from build123d import *

# Parameters (mm, degrees)
SKETCH1_W           = 25
SKETCH1_H           = 23.9
SKETCH1_R           = 1
BOSS_EXTRUDE1_DEPTH = 0.95
SKETCH2_W           = 7.5
SKETCH2_H           = 5
BOSS_EXTRUDE2_DEPTH = 1.45
SKETCH3_W           = 8
SKETCH3_H           = 8
BOSS_EXTRUDE3_DEPTH = 4.4
SKETCH4_W           = 8
SKETCH4_H           = 8
SKETCH4_R           = 3.75
CUT_EXTRUDE1_DEPTH  = 0.9
SKETCH5_R           = 2.775
CUT_EXTRUDE2_DEPTH  = 3.9
BOSS_EXTRUDE4_DEPTH = 6
BOSS_EXTRUDE5_DEPTH = 2.8


with BuildPart() as part:
    # Sketch1 → Boss-Extrude1 (new body)
    with BuildSketch(Plane.XY):
        with Locations((12.5, 11.95)):
            Rectangle(SKETCH1_W, SKETCH1_H)
        with Locations((23, 9.35)):
            Circle(SKETCH1_R, mode=Mode.SUBTRACT)
        with Locations((2, 9.35)):
            Circle(SKETCH1_R, mode=Mode.SUBTRACT)
        with Locations((23, 21.85)):
            Circle(SKETCH1_R, mode=Mode.SUBTRACT)
        with Locations((2, 21.85)):
            Circle(SKETCH1_R, mode=Mode.SUBTRACT)
    extrude(amount=BOSS_EXTRUDE1_DEPTH)

    # Sketch2 → Boss-Extrude2 (add)
    with BuildSketch(Plane.XY.offset(0.95)):
        with Locations((12.5, 19.2)):
            Rectangle(SKETCH2_W, SKETCH2_H)
    extrude(amount=BOSS_EXTRUDE2_DEPTH)

    # Sketch3 → Boss-Extrude3 (add)
    with BuildSketch(Plane.XY.offset(0.95)):
        with Locations((12.5, 9.1)):
            Rectangle(SKETCH3_W, SKETCH3_H)
    extrude(amount=BOSS_EXTRUDE3_DEPTH)

    # Sketch4 → Cut-Extrude1 (cut)
    with BuildSketch(Plane.XY.offset(5.35)):
        with Locations((12.5, 9.1)):
            Rectangle(SKETCH4_W, SKETCH4_H)
        with Locations((12.5, 9.1)):
            Circle(SKETCH4_R, mode=Mode.SUBTRACT)
    extrude(amount=-CUT_EXTRUDE1_DEPTH, mode=Mode.SUBTRACT)

    # Sketch5 → Cut-Extrude2 (cut)
    with BuildSketch(Plane.XY.offset(5.35)):
        with Locations((12.5, 9.1)):
            Circle(SKETCH5_R)
    extrude(amount=-CUT_EXTRUDE2_DEPTH, mode=Mode.SUBTRACT)

    # Sketch12 → Boss-Extrude4 (add)
    with BuildSketch(Plane(origin=(15.5, 0, 0), x_dir=(0, 0, -1), z_dir=(1, 0, 0))):
        Polygon((-2.4, 16.7), (-2.3, 16.7), (-0.95, 13.1), (-1.05, 13.1), align=None)
    extrude(amount=-BOSS_EXTRUDE4_DEPTH)

    # Sketch13 → Boss-Extrude5 (add)
    with BuildSketch(Plane(origin=(0, 0, 0), x_dir=(-1, 0, 0), z_dir=(0, 0, -1))):
        Polygon((-1.4, 5.6), (-12.5, 5.6), (-23.6, 5.6), (-23.6, 0.2), (-1.4, 0.2), align=None)
    extrude(amount=BOSS_EXTRUDE5_DEPTH)


solid = part.part
Build history of the part. All positions in model axes, mm. A direction names the side the tool comes from. Round coordinates to 2 decimals unless told otherwise and drop trailing zeros. Loops run counter-clockwise (first coordinate to the right, second up) from the corner with the lowest first, then second, coordinate; pieces in that order, holes last. Notation, with made-up numbers: (-12, -17.75) -> (-5, -17.75) arc R20 ccw to (-5, -10.75) -> close; hole circle Ø7 at (37, 7.25). An arc over 180 degrees is marked (long way). One line per item, written item: value. Start each with the question number.
Q1. Cut at B-B on x = 23. List the corners of the cut face in (y, z), plus the area to 3 significant figures.
Q2. Probe line 1 along Y through (x, z) = (23, 0.45); line 2 along Y through (x, z) = (12.5, 2.7) (3 decimals); line 3 along X through (y, z) = (9.25, 3.75). List the from-to ranges inside material, lowest first.
Q3. Cut at A-A on x = 12.5. List the corners of the cut face in (y, z) (3 decimals).
Q4. Cut at D-D on z = 3.5. List the corners of the cut face in (x, y) (3 decimals), plus the area to 3 significant figures.
Q5. 3-axis set-ups, long thin cutter, end or side, ignore diameter. For faces 1 (the face through (12, 5.1, 3)), 2 (the face through (12, 9, 1.45)), 3 (the face through (1.4, 3, -1)): which of +Z, -Z, +X, -X, +Y, -Y reach the whole face in a straight line?
Q6. Cut at C-C on y = 14.75. List the corners of the cut face in (x, z), plus the area to 4 significant figures.
Q7. Drop flat-ended pins along their axis: pin 1 Ø1.6 at (x, z) = (14, 2) entering from +Y; pin 2 Ø2 at (y, z) = (8, 2.5) entering from +X; pin 3 Ø1 at (y, z) = (9.5, 3.5) entering from -X. Give the stop position or say it passes through.
Q8. Two-plate mould, pull along Z, no slides. Class faces 4 (the face through (12, 16.7, 2)), 5 (the face through (13, 3, -2.8)), 6 (the face through (12, 12, 5.35)): released by +Z, released by -Z, zero draft, split by the parting line, or undercut.
Computed:
1. outline: (0, 0) -> (0.2, 0) -> (0.2, -2.8) -> (5.6, -2.8) -> (5.6, 0) -> (8.35, 0) -> (8.35, 0.95) -> (0, 0.95) -> close; (10.35, 0) -> (20.85, 0) -> (20.85, 0.95) -> (10.35, 0.95) -> close; (22.85, 0) -> (23.9, 0) -> (23.9, 0.95) -> (22.85, 0.95) -> close
1. area: 34.0 mm²
2. line 1: 0 to 8.35, 10.35 to 20.85, 22.85 to 23.9
2. line 2: 5.1 to 6.325, 11.875 to 13.1
2. line 3: 8.5 to 9.73, 15.27 to 16.5
3. outline: (0, 0) -> (0.2, 0) -> (0.2, -2.8) -> (5.6, -2.8) -> (5.6, 0) -> (23.9, 0) -> (23.9, 0.95) -> (21.7, 0.95) -> (21.7, 2.4) -> (16.7, 2.4) -> (13.1, 1.05) -> (13.1, 4.45) -> (12.85, 4.45) -> (12.85, 5.35) -> (11.875, 5.35) -> (11.875, 1.45) -> (6.325, 1.45) -> (6.325, 5.35) -> (5.35, 5.35) -> (5.35, 4.45) -> (5.1, 4.45) -> (5.1, 0.95) -> (0, 0.95) -> close; hole (13.1, 0.95) -> (16.7, 0.95) -> (16.7, 2.3) -> close
4. outline: (8.5, 5.1) -> (16.5, 5.1) -> (16.5, 13.1) -> (8.5, 13.1) -> close; hole circle Ø5.55 at (12.5, 9.1)
4. area: 39.8 mm²
5. face 1: +Z, +X, -X, -Y
5. face 2: +Z
5. face 3: -Z, -X, +Y, -Y
6. outline: (0, 0) -> (25, 0) -> (25, 0.95) -> (0, 0.95) -> close; (9.5, 1.57) -> (15.5, 1.57) -> (15.5, 1.67) -> (9.5, 1.67) -> close
6. area: 24.35 mm²
7. pin 1: y = 21.7
7. pin 2: x = 16.5
7. pin 3: x = 8.5
8. face 4: undercut
8. face 5: released by -Z
8. face 6: released by +Z
